```python
from build123d import *

# Parameters (mm, degrees)
BOX_W        = 70.104
BOX_H        = 9.3472
BOX_DEPTH    = 15.494
BOX001_W     = 66.04
BOX001_H     = 1.8669
BOX001_DEPTH = 7.493
BOX002_W     = 1.524
BOX002_H     = 9.3472
BOX002_DEPTH = 4.572
BOX003_W     = 1.524
BOX003_H     = 9.3472
BOX003_DEPTH = 4.572
FILLET_R     = 0.5
FILLET001_R  = 0.5
FILLET002_R  = 0.5
FILLET003_R  = 0.5
FILLET004_R  = 0.5
FILLET005_R  = 0.5
FILLET006_R  = 0.5
FILLET007_R  = 0.5
FILLET008_R  = 0.5
FILLET009_R  = 0.5
BOX004_W     = 64.516
BOX004_H     = 9.3472
BOX004_DEPTH = 1.524
BOX005_W     = 1.016
BOX005_H     = 0.762
BOX005_DEPTH = 13
BOX006_W     = 1.016
BOX006_H     = 0.762
BOX006_DEPTH = 9


with BuildPart() as part:
    # Box → Box (join)
    with BuildSketch(Plane(origin=(-35.052, -4.6736, 0), x_dir=(1, 0, 0), z_dir=(0, 0, 1))):
        with Locations((35.052, 4.6736)):
            Rectangle(BOX_W, BOX_H)
    extrude(amount=BOX_DEPTH)

    # Box001 → Box001 (cut)
    with BuildSketch(Plane(origin=(-33.02, -0.93345, 8.01), x_dir=(1, 0, 0), z_dir=(0, 0, 1))):
        with Locations((33.02, 0.93345)):
            Rectangle(BOX001_W, BOX001_H)
    extrude(amount=BOX001_DEPTH, mode=Mode.SUBTRACT)

    # Box002 → Box002 (cut)
    with BuildSketch(Plane(origin=(-35.052, -4.6736, 0), x_dir=(1, 0, 0), z_dir=(0, 0, 1))):
        with Locations((0.762, 4.6736)):
            Rectangle(BOX002_W, BOX002_H)
    extrude(amount=BOX002_DEPTH, mode=Mode.SUBTRACT)

    # Box003 → Box003 (cut)
    with BuildSketch(Plane(origin=(33.53, -4.6736, 0), x_dir=(1, 0, 0), z_dir=(0, 0, 1))):
        with Locations((0.762, 4.6736)):
            Rectangle(BOX003_W, BOX003_H)
    extrude(amount=BOX003_DEPTH, mode=Mode.SUBTRACT)

    # Fillet
    fillet_edges = [part.edges().sort_by_distance(p)[0] for p in [
        (-35.052, -4.6736, 10.033),
    ]]
    fillet(fillet_edges, radius=FILLET_R)

    # Fillet001
    fillet001_edges = [part.edges().sort_by_distance(p)[0] for p in [
        (-35.052, 4.6736, 10.033),
    ]]
    fillet(fillet001_edges, radius=FILLET001_R)

    # Fillet002
    fillet002_edges = [part.edges().sort_by_distance(p)[0] for p in [
        (-33.528, -4.6736, 2.286),
    ]]
    fillet(fillet002_edges, radius=FILLET002_R)

    # Fillet003
    fillet003_edges = [part.edges().sort_by_distance(p)[0] for p in [
        (-33.528, 4.6736, 2.286),
    ]]
    fillet(fillet003_edges, radius=FILLET003_R)

    # Fillet004
    fillet004_edges = [part.edges().sort_by_distance(p)[0] for p in [
        (33.53, -4.6736, 2.286),
    ]]
    fillet(fillet004_edges, radius=FILLET004_R)

    # Fillet005
    fillet005_edges = [part.edges().sort_by_distance(p)[0] for p in [
        (35.052, -4.6736, 10.033),
    ]]
    fillet(fillet005_edges, radius=FILLET005_R)

    # Fillet006
    fillet006_edges = [part.edges().sort_by_distance(p)[0] for p in [
        (33.53, 4.6736, 2.286),
    ]]
    fillet(fillet006_edges, radius=FILLET006_R)

    # Fillet007
    fillet007_edges = [part.edges().sort_by_distance(p)[0] for p in [
        (35.052, 4.6736, 10.033),
    ]]
    fillet(fillet007_edges, radius=FILLET007_R)

    # Fillet008
    fillet008_edges = [part.edges().sort_by_distance(p)[0] for p in [
        (0, -0.93345, 15.494),
    ]]
    fillet(fillet008_edges, radius=FILLET008_R)

    # Fillet009
    fillet009_edges = [part.edges().sort_by_distance(p)[0] for p in [
        (0, 0.93345, 15.494),
    ]]
    fillet(fillet009_edges, radius=FILLET009_R)

    # Box004 → Box004 (cut)
    with BuildSketch(Plane(origin=(-32.258, -4.6736, 0), x_dir=(1, 0, 0), z_dir=(0, 0, 1))):
        with Locations((32.258, 4.6736)):
            Rectangle(BOX004_W, BOX004_H)
    extrude(amount=BOX004_DEPTH, mode=Mode.SUBTRACT)

    # Box005 → Box005 (cut)
    with BuildSketch(Plane(origin=(-0.508, -2.9337, 0), x_dir=(1, 0, 0), z_dir=(0, 0, 1))):
        with Locations((0.508, 0.381)):
            Rectangle(BOX005_W, BOX005_H)
    extrude(amount=BOX005_DEPTH, mode=Mode.SUBTRACT)

    # Box006 → Box006 (cut)
    with BuildSketch(Plane(origin=(-0.508, 2.1717, 0), x_dir=(1, 0, 0), z_dir=(0, 0, 1))):
        with Locations((0.508, 0.381)):
            Rectangle(BOX006_W, BOX006_H)
    extrude(amount=BOX006_DEPTH, mode=Mode.SUBTRACT)


solid = part.part
```
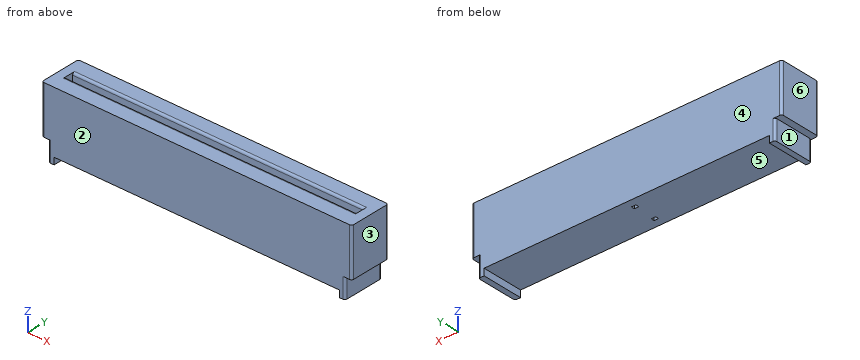
Work out the finished part from the listing and answer in its coordinate system (mm). Face numbers are marked on the shaded views. A direction names the side the tool comes from. Give positions to 0.01 mm unless a question says otherwise; leave off trailing zeros. Order: outer loops, then holes, each group sorted by start corner. A loop starts at its lowest first (then second) coordinate and runs counter-clockwise, first axis right, second up.
1. Each of these flat-tipped pins is pushed along its axis until it touches: P1, Ø0.5, axis at y = 2.5, z = 0.5, coming from the -X side; P2, Ø0.6, axis at x = 7, y = 0.5, coming from the +Z side; P3, Ø0.8, axis at x = 0, y = -2.5, coming from the -Z side. Where does it stop, or does it pass through?
Result sheet:
P1: stops at x = -33.53
P2: stops at z = 8.01
P3: stops at z = 1.52
2. The mould has two halves that part along X. Classify the marked faces 3, 4, 5 and 6: released by +X, released by -X, zero draft, split by the parting line, or undercut.
Result sheet:
face 3: released by +X
face 4: zero draft
face 5: undercut
face 6: released by -X
3. Section D-D, the plane x = 8.5 is taken. Determine the outline of the cut face in (y, z).
Result sheet:
outline: (-4.67, 1.52) - (4.67, 1.52) - (4.67, 15.49) - (1.43, 15.49) arc R0.5 ccw to (0.93, 14.99) - (0.93, 8.01) - (-0.93, 8.01) - (-0.93, 14.99) arc R0.5 ccw to (-1.43, 15.49) - (-4.67, 15.49) - close
4. Section C-C, the plane z = 14 is taken. Determine the outline of the cut face in (x, y).
Result sheet:
outline: (-35.05, -4.17) arc R0.5 ccw to (-34.55, -4.67) - (34.55, -4.67) arc R0.5 ccw to (35.05, -4.17) - (35.05, 4.17) arc R0.5 ccw to (34.55, 4.67) - (-34.55, 4.67) arc R0.5 ccw to (-35.05, 4.17) - close; hole (-33.02, -0.93) - (33.02, -0.93) - (33.02, 0.93) - (-33.02, 0.93) - close
5. For the marked faces 1 and 2, determine the directions among +Z, -Z, +X, -X, +Y, -Y from which every point of the face is accessible in a straight line to the end or side of a thin tool.
Result sheet:
face 1: -Z, -X, +Y, -Y
face 2: +Z, -Z, +X, -X, -Y
6. Section B-B, the plane y = -0.25 is taken. Determine the outline of the cut face in (x, z), and give its area (3 significant figures).
Result sheet:
outline: (-35.05, 4.57) - (-33.53, 4.57) - (-33.53, 0) - (-32.26, 0) - (-32.26, 1.52) - (32.26, 1.52) - (32.26, 0) - (33.53, 0) - (33.53, 4.57) - (35.05, 4.57) - (35.05, 15.49) - (33.02, 15.49) - (33.02, 8.01) - (-33.02, 8.01) - (-33.02, 15.49) - (-35.05, 15.49) - close
area: 480 mm2
7. Straight lines are drawn through the part: L1, parallel to Y at x = 31, z = 10.5; L2, parallel to X at y = -0.25, z = 12; L3, parallel to Z at x = 11, y = 2.25. For each, find the intervals that lie inside material, in ascending order.
Result sheet:
L1: y = -4.67 to -0.93, 0.93 to 4.67
L2: x = -35.05 to -33.02, 33.02 to 35.05
L3: z = 1.52 to 15.49
8. Section A-A, the plane z = 3.75 is taken. Determine the outline of the cut face in (x, y), and give its area (3 significant figures).
Result sheet:
outline: (-33.53, -4.17) arc R0.5 ccw to (-33.03, -4.67) - (33.03, -4.67) arc R0.5 ccw to (33.53, -4.17) - (33.53, 4.17) arc R0.5 ccw to (33.03, 4.67) - (-33.03, 4.67) arc R0.5 ccw to (-33.53, 4.17) - close; hole (-0.51, -2.93) - (0.51, -2.93) - (0.51, -2.17) - (-0.51, -2.17) - close; hole (-0.51, 2.17) - (0.51, 2.17) - (0.51, 2.93) - (-0.51, 2.93) - close
area: 625 mm2
